Can you work these out from the model? Positions are in its coordinate system, mm. Face numbers are marked on the shaded views. A direction names the side the tool comes from. Round coordinates to 2 decimals unless told otherwise and drop trailing zeros. Loops run counter-clockwise (first coordinate to the right, second up) from the corner with the lowest first, then second, coordinate; pieces in that order, holes last.
(1) I want a section at B-B on x = -22.65. Write out the boundary of the cut face in (y, z).
(2) Which directions (+Z, -Z, +X, -X, +Y, -Y) give clear straight access to the entire face, cutting with the end or side of a thin tool? Please do the marked faces 4, 5, 6 and 7.
(3) I want a section at A-A on z = 42. Write out the boundary of the cut face in (x, y), plus the area to 3 significant figures.
(4) If I drill on line 1 along Y through (x, z) = (0, 2.25); line 2 along Z through (x, y) = (5, -2); line 3 along Y through (x, z) = (6, 6), over which ranges is the centre line in solid material (lowest first)?
(5) Will these pins go through, and if not, where does the flat tip stop? pin 1 Ø6 at (y, z) = (0, 38.5) entering from +X; pin 2 Ø4 at (y, z) = (-4.5, 8) entering from +X; pin 3 Ø2 at (x, z) = (-9.5, 52) entering from +Y; pin 4 Ø4 at (x, y) = (-22.65, 0) entering from -Z.
(6) Thinking about a two-plate mould opening in Z: for the marked faces 1, 2 and 3, which applies, released by +Z, released by -Z, zero draft, split by the parting line, or undercut?
from build123d import *

# Parameters (mm, degrees)
SKETCH1_R               = 25.65
SKETCH1_R_2             = 1.45
BOSS_EXTRUDE1_DEPTH     = 10
CUT_EXTRUDE2_DEPTH      = 38.627715849
CUT_EXTRUDE2_DEPTH_BACK = 7.4
SKETCH3_R               = 0.95
CUT_EXTRUDE3_DEPTH      = 15
BOSS_EXTRUDE2_DEPTH     = 41.11
BOSS_EXTRUDE3_DEPTH     = 10
SKETCH6_R               = 0.95
CUT_EXTRUDE4_DEPTH      = 15
FILLET1_R               = 4
BOSS_EXTRUDE4_DEPTH     = 51.11
FILLET2_R               = 4
FILLET3_R               = 3


with BuildPart() as part:
    # Sketch1 → Boss-Extrude1 (new body)
    with BuildSketch(Plane.XY):
        Circle(SKETCH1_R)
        with Locations((0, -22.65)):
            Circle(SKETCH1_R_2, mode=Mode.SUBTRACT)
        with Locations((22.65, 0)):
            Circle(SKETCH1_R_2, mode=Mode.SUBTRACT)
        with Locations((0, 22.65)):
            Circle(SKETCH1_R_2, mode=Mode.SUBTRACT)
        with Locations((-22.65, 0)):
            Circle(SKETCH1_R_2, mode=Mode.SUBTRACT)
    extrude(amount=BOSS_EXTRUDE1_DEPTH)

    # Sketch2 → Cut-Extrude2 (cut, two sides: drawn at the far end of the back side and taken through both)
    with BuildSketch(Plane.XY.offset(10).offset(-CUT_EXTRUDE2_DEPTH_BACK)):
        Polygon((102.061719716, 116.734185426), (9.251139978, 23.923605688), (1.028840367, 15.701306076), (15.701306076, 1.028840367), (23.923605688, 9.251139978), (116.734185426, 102.061719716), (302.355344902, 287.682879192), (287.682879192, 302.355344902), align=None)
    extrude(amount=CUT_EXTRUDE2_DEPTH + CUT_EXTRUDE2_DEPTH_BACK, mode=Mode.SUBTRACT)

    # Sketch3 → Cut-Extrude3 (cut)
    with BuildSketch(Plane(origin=(8.365073221, 8.365073221, 0), x_dir=(0, 0, -1), z_dir=(0.7071067811865477, 0.7071067811865475, 0))):
        with Locations(Location((-5.74, 4.95, 0), (0, 0, 90))):
            Circle(SKETCH3_R)
        with Locations(Location((-5.74, -4.95, 0), (0, 0, 270))):
            Circle(SKETCH3_R)
    extrude(amount=-CUT_EXTRUDE3_DEPTH, mode=Mode.SUBTRACT)

    # Sketch4 → Boss-Extrude2 (add)
    with BuildSketch(Plane.XY.offset(10)):
        Polygon((-3.920907102, 20.651053545), (1.028840367, 15.701306076), (-9.577761351, 5.094704358), (-14.527508819, 10.044451827), align=None)
        Polygon((15.701306076, 1.028840367), (5.094704358, -9.577761351), (10.044451827, -14.527508819), (20.651053545, -3.920907102), align=None)
    extrude(amount=BOSS_EXTRUDE2_DEPTH)

    # Sketch5 → Boss-Extrude3 (add)
    with BuildSketch(Plane.XY.offset(51.11)):
        Polygon((-3.920907102, 20.651053545), (-14.527508819, 10.044451827), (10.044451827, -14.527508819), (20.651053545, -3.920907102), align=None)
    extrude(amount=BOSS_EXTRUDE3_DEPTH)

    # Sketch6 → Cut-Extrude4 (cut)
    with BuildSketch(Plane(origin=(8.365073221, 8.365073221, 0), x_dir=(0, 0, -1), z_dir=(0.7071067811865471, 0.707106781186548, 0))):
        with Locations(Location((-5.74, -4.95, 0), (0, 0, 270))):
            Circle(SKETCH6_R)
        with Locations(Location((-5.74, 4.95, 0), (0, 0, 90))):
            Circle(SKETCH6_R)
        with Locations(Location((-54.37, -4.95, 0), (0, 0, 270))):
            Circle(SKETCH6_R)
        with Locations(Location((-54.37, 4.95, 0), (0, 0, 270))):
            Circle(SKETCH6_R)
    extrude(amount=-CUT_EXTRUDE4_DEPTH, mode=Mode.SUBTRACT)

    # Fillet1
    fillet1_edges = [part.edges().sort_by_distance(p)[0] for p in [
        (-9.224207961, 15.347752686, 10),
        (-12.052635085, 7.569578093, 10),
        (7.569578093, -12.052635085, 10),
        (15.347752686, -9.224207961, 10),
    ]]
    fillet(fillet1_edges, radius=FILLET1_R)

    # Sketch7 → Boss-Extrude4 (add)
    with BuildSketch(Plane.XY.offset(10)):
        with BuildLine():
            Line((6.41546388, 24.834740248), (-0.844564963, 17.574711406))
            Line((-0.844564963, 17.574711406), (1.028840367, 15.701306076))
            Line((1.028840367, 15.701306076), (9.251139978, 23.923605688))
            ThreePointArc((9.251139978, 23.923605688), (7.846538132, 24.420367306), (6.41546388, 24.834740248))
        make_face()
        with BuildLine():
            Line((17.574711406, -0.844564963), (24.834740248, 6.41546388))
            ThreePointArc((24.834740248, 6.41546388), (24.420367306, 7.846538132), (23.923605688, 9.251139978))
            Line((23.923605688, 9.251139978), (15.701306076, 1.028840367))
            Line((15.701306076, 1.028840367), (17.574711406, -0.844564963))
        make_face()
    extrude(amount=BOSS_EXTRUDE4_DEPTH)

    # Fillet2
    fillet2_edges = [part.edges().sort_by_distance(p)[0] for p in [
        (-0.844564963, 17.574711406, 35.555),
        (17.574711406, -0.844564963, 35.555),
    ]]
    fillet(fillet2_edges, radius=FILLET2_R)

    # Fillet3
    fillet3_edges = [part.edges().sort_by_distance(p)[0] for p in [
        (-9.224207961, 15.347752686, 61.11),
        (15.347752686, -9.224207961, 61.11),
    ]]
    fillet(fillet3_edges, radius=FILLET3_R)


solid = part.part
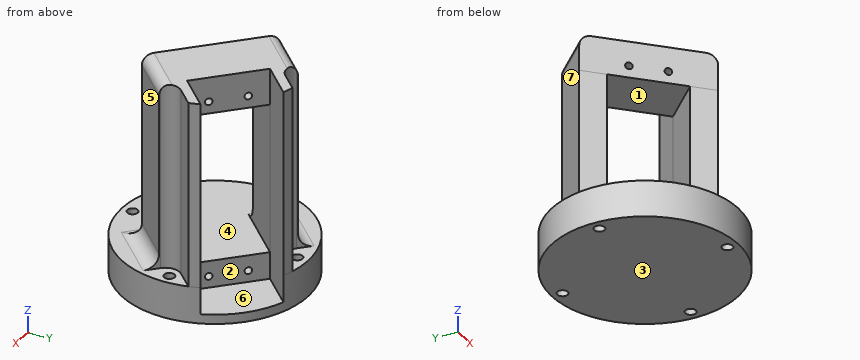
Filled sheet:
1. outline: (-12.04, 0) - (-1.45, 0) - (-1.45, 10) - (-12.04, 10) - close; (1.45, 0) - (12.04, 0) - (12.04, 10) - (1.45, 10) - close
2. face 4: none
2. face 5: +Z, +X, -Y
2. face 6: +Z
2. face 7: +Z, -X, +Y
3. outline: (-14.53, 10.04) - (-9.58, 5.09) - (9.25, 23.92) arc R25.65 ccw to (6.42, 24.83) - (1.98, 20.4) arc R4 cw to (-3.67, 20.4) - (-3.92, 20.65) - close; (5.09, -9.58) - (10.04, -14.53) - (20.65, -3.92) - (20.4, -3.67) arc R4 cw to (20.4, 1.98) - (24.83, 6.42) arc R25.65 ccw to (23.92, 9.25) - close
3. area: 275 mm2
4. line 1: y = -25.65 to -24.1, -21.2 to 21.2, 24.1 to 25.65
4. line 2: z = 0 to 4.79, 6.69 to 10, 51.11 to 53.42, 55.32 to 61.11
4. line 3: y = -24.94 to -2.29, 0.29 to 10.73, 20.67 to 24.94
5. pin 1: stops at x = 21.42
5. pin 2: stops at x = 25.53
5. pin 3: stops at y = 16.07
5. pin 4: stops at z = 0
6. face 1: undercut
6. face 2: zero draft
6. face 3: released by -Z
